Autodesk Inventor part; units mm, degrees
ref_plane "YZ Plane" through (0, 0, 0) normal (1, 0, 0) x (0, 1, 0)
ref_plane "XZ Plane" through (0, 0, 0) normal (0, 1, 0) x (-1, 0, 0)
ref_plane "XY Plane" through (0, 0, 0) normal (0, 0, 1) x (1, 0, 0)
sketch "Sketch1" plane through (0, 0, 0) normal (0, 1, 0) x (-1, 0, 0)
  line L0 (0, 0) -> (75, 0)
  line L1 (77, -2) -> (77, -75)
  line L2 (75, -77) -> (2, -77)
  line L3 (0, -75) -> (0, 0)
  line L4 (0, 0) -> (0, -8.5)
  line L5 (6, -8.5) -> (8.5, -8.5)
  line L6 (8.5, -48.5) -> (8.5, -68.5)
  circle A0 centre (8.5, -8.5) radius 2.5
  circle A1 centre (8.5, -28.5) radius 2.5
  circle A2 centre (8.5, -48.5) radius 2.5
  circle A3 centre (8.5, -68.5) radius 2.5
  line L7 (68.5, -28.5) -> (68.5, -48.5)
  line L8 (68.5, -48.5) -> (68.5, -68.5)
  line L9 (68.5, -68.5) -> (38.5, -68.5)
  circle A4 centre (38.5, -8.5) radius 2.5
  circle A5 centre (68.5, -8.5) radius 2.5
  circle A6 centre (68.5, -28.5) radius 2.5
  circle A7 centre (68.5, -48.5) radius 2.5
  circle A8 centre (68.5, -68.5) radius 2.5
  circle A9 centre (38.5, -68.5) radius 2.5
  line L10 (77, 0) -> (58.5, 0)
  line L11 (58.5, -18.5) -> (61, -18.5)
  line L12 (77, -18.5) -> (77, 0)
  line L13 (2, 0) -> (18.5, 0)
  line L14 (18.5, -8.5) -> (18.5, -18.5)
  line L15 (18.5, -18.5) -> (0, -18.5)
  line L16 (0, -18.5) -> (0, -2)
  line L17 (0, -77) -> (18.5, -77)
  line L18 (18.5, -61) -> (18.5, -58.5)
  line L19 (0, -58.5) -> (0, -77)
  circle A10 centre (58.5, -18.5) radius 2.5
  circle A11 centre (18.5, -18.5) radius 2.5
  circle A12 centre (18.5, -58.5) radius 2.5
  circle A13 centre (58.5, -58.5) radius 2.5
  line L20 (18.5, -18.5) -> (28.5, -18.5)
  line L21 (58.5, -58.5) -> (48.5, -58.5)
  circle A14 centre (28.5, -18.5) radius 2.5
  circle A15 centre (48.5, -18.5) radius 2.5
  circle A16 centre (48.5, -58.5) radius 2.5
  circle A17 centre (28.5, -58.5) radius 2.5
  line L22 (58.5, -38.5) -> (48.5, -38.5)
  line L23 (28.5, -38.5) -> (18.5, -38.5)
  circle A18 centre (58.5, -38.5) radius 2.5
  circle A19 centre (48.5, -38.5) radius 2.5
  circle A20 centre (28.5, -38.5) radius 2.5
  circle A21 centre (18.5, -38.5) radius 2.5
  circle A22 centre (38.5, -28.5) radius 2.5
  circle A23 centre (38.5, -38.5) radius 2.5
  line L24 (28.5, -58.5) -> (28.5, -38.5)
  circle A24 centre (38.5, -48.5) radius 2.5
  line L25 (36, -48.5) -> (36, -38.5)
  line L26 (41, -38.5) -> (41, -48.5)
  arc A25 (77, -2) -> (75, 0) centre (75, -2) ccw
  arc A26 (75, -77) -> (77, -75) centre (75, -75) ccw
  arc A27 (0, -75) -> (2, -77) centre (2, -75) ccw
  arc A28 (2, 0) -> (0, -2) centre (2, -2) ccw
  line L27 (68.5, -8.5) -> (68.5, -11)
  line L28 (68.5, -26) -> (68.5, -28.5)
  line L29 (58.5, 0) -> (58.5, -8.5)
  line L30 (58.5, -16) -> (58.5, -18.5)
  line L31 (38.5, -8.5) -> (41, -8.5)
  line L32 (66, -8.5) -> (68.5, -8.5)
  line L33 (58.5, -18.5) -> (58.5, -21)
  line L34 (58.5, -36) -> (58.5, -38.5)
  line L35 (58.5, -18.5) -> (56, -18.5)
  line L36 (51, -18.5) -> (48.5, -18.5)
  line L37 (48.5, -18.5) -> (46.7322, -20.2678)
  line L38 (40.2678, -26.7322) -> (28.5, -38.5)
  line L39 (28.5, -18.5) -> (40.2678, -30.2678)
  line L40 (46.7322, -36.7322) -> (48.5, -38.5)
  line L41 (48.5, -38.5) -> (46, -38.5)
  line L42 (41, -38.5) -> (28.5, -38.5)
  line L43 (48.5, -38.5) -> (46.7322, -40.2678)
  line L44 (41, -46) -> (36.7322, -50.2678)
  line L45 (30.2678, -56.7322) -> (28.5, -58.5)
  line L46 (48.5, -58.5) -> (36, -46)
  line L47 (30.2678, -40.2678) -> (28.5, -38.5)
  line L48 (18.5, -58.5) -> (21, -58.5)
  line L49 (26, -58.5) -> (28.5, -58.5)
  line L50 (18.5, -58.5) -> (16, -58.5)
  line L51 (8.5, -58.5) -> (0, -58.5)
  line L52 (8.5, -28.5) -> (8.5, -31)
  line L53 (8.5, -46) -> (8.5, -48.5)
  line L54 (8.5, -8.5) -> (8.5, -11)
  line L55 (8.5, -26) -> (8.5, -28.5)
  line L56 (8.5, -8.5) -> (11, -8.5)
  line L57 (18.5, -8.5) -> (38.5, -8.5)
  line L58 (28.5, -38.5) -> (28.5, -36)
  line L59 (28.5, -21) -> (28.5, -18.5)
  point P0 (77, -77)
  dimension "d9" = 5
  dimension "d15" = 5
  dimension "d17" = 5
  dimension "d29" = 5
  dimension "d32" = 5
  dimension "d0" = 77
  dimension "d1" = 77
  dimension "d2" = 8.5
  dimension "d3" = 8.5
  dimension "d4" = 20
  dimension "d5" = 20
  dimension "d6" = 20
  dimension "d7" = 5
  dimension "d8" = 5
  dimension "d10" = 5
  dimension "d11" = 30
  dimension "d12" = 30
  dimension "d13" = 20
  dimension "d14" = 20
  dimension "d16" = 5
  dimension "d18" = 18.5
  dimension "d19" = 18.5
  dimension "d20" = 18.5
  dimension "d21" = 18.5
  dimension "d22" = 18.5
  dimension "d23" = 18.5
  dimension "d24" = 5
  dimension "d25" = 5
  dimension "d26" = 10
  dimension "d27" = 10
  dimension "d28" = 10
  dimension "d30" = 5
  dimension "d31" = 20
  dimension "d33" = 5
  dimension "d34" = 5
  dimension "d35" = 2
  dimension "d36" = 2
extrude "Extrusion1" add sketch "Sketch1" along normal blind 6 contours L0 A25 L1 A26 L2 A27 L3 A28
sketch "Sketch2" plane through (0, 6, 0) normal (0, 1, 0) x (1, 0, 0)
  line L0 (0, 0) -> (-23.5, 0)
  line L1 (-23.5, 0) -> (-23.5, 23.5)
  line L2 (-23.5, 23.5) -> (0, 23.5)
  line L3 (0, 23.5) -> (0, 0)
  line L4 (-77, 75) -> (-77, 2)
  line L5 (-77, 67.2397) -> (-77, 80.0778)
  line L6 (-2, 77) -> (-75, 77)
  line L7 (-67.8517, 77) -> (-77, 77)
  line L8 (-77, 77) -> (-53.5, 77)
  line L9 (-53.5, 77) -> (-53.5, 53.5)
  line L10 (-53.5, 53.5) -> (-77, 53.5)
  line L11 (-77, 53.5) -> (-77, 77)
  line L12 (-51.5, 53.5) -> (-25.5, 53.5)
  line L13 (-23.5, 51.5) -> (-23.5, 25.5)
  line L14 (-25.5, 23.5) -> (-51.5, 23.5)
  line L15 (-53.5, 25.5) -> (-53.5, 51.5)
  arc A0 (-53.5, 25.5) -> (-51.5, 23.5) centre (-51.5, 25.5) ccw
  arc A1 (-25.5, 23.5) -> (-23.5, 25.5) centre (-25.5, 25.5) ccw
  arc A2 (-23.5, 51.5) -> (-25.5, 53.5) centre (-25.5, 51.5) ccw
  arc A3 (-51.5, 53.5) -> (-53.5, 51.5) centre (-51.5, 51.5) ccw
  dimension "d39" = 23.5
  dimension "d40" = 23.5
  dimension "d41" = 23.5
  dimension "d42" = 23.5
  dimension "d43" = 2
extrude "Extrusion2" cut sketch "Sketch2" against normal blind 1 contours L12 A2 L13 A1 L14 A0 L15 A3
sketch "Sketch3" plane through (0, 0, 0) normal (0, -1, 0) x (1, 0, 0)
  line L0 (-51.5, -53.5) -> (-25.5, -53.5)
  line L1 (-53.5, -25.5) -> (-53.5, -51.5)
  line L2 (-25.5, -23.5) -> (-51.5, -23.5)
  line L3 (-23.5, -51.5) -> (-23.5, -25.5)
  line L4 (-53.5, -53.5) -> (-23.5, -53.5)
  line L5 (-23.5, -53.5) -> (-23.5, -38.5)
  line L6 (-53.5, -38.5) -> (-23.5, -38.5)
  line L7 (-53.5, -38.5) -> (-53.5, -53.5)
  point P0 (0, 0)
extrude "Extrusion3" add sketch "Sketch3" along normal blind 15
sketch "Sketch4" plane through (-23.5, 0, -53.5) normal (0, 0, -1) x (-1, 0, 0)
  line L0 (2.5, 0) -> (0, 0)
  line L1 (0, 0) -> (0, -15)
  line L2 (0, -8) -> (15, -8)
  line L3 (30, 0) -> (30, -15)
  circle A0 centre (15, -8) radius 4
  line L4 (0, 0) -> (0, -15)
  line L5 (0, -8) -> (0, -15)
  line L6 (30, -15) -> (0, -15)
  point P0 (-23.5, 0)
  dimension "d49" = 15
  dimension "d50" = 8
  dimension "d53" = 7
extrude "Extrusion4" cut sketch "Sketch4" against normal blind 22
sketch "Sketch5" plane through (0, 6, 0) normal (0, 1, 0) x (1, 0, 0)
  arc A0 (-25.5, 23.5) -> (-23.5, 25.5) centre (-25.5, 25.5) ccw
  line L0 (-25.5, 23.5) -> (-51.5, 23.5)
  arc A1 (-53.5, 25.5) -> (-51.5, 23.5) centre (-51.5, 25.5) ccw
  line L1 (-53.5, 25.5) -> (-53.5, 51.5)
  arc A2 (-51.5, 53.5) -> (-53.5, 51.5) centre (-51.5, 51.5) ccw
  line L2 (-51.5, 53.5) -> (-25.5, 53.5)
  arc A3 (-23.5, 51.5) -> (-25.5, 53.5) centre (-25.5, 51.5) ccw
  line L3 (-23.5, 51.5) -> (-23.5, 25.5)
  arc A4 (0, 75) -> (-2, 77) centre (-2, 75) ccw
  line L4 (-2, 77) -> (-75, 77)
  arc A5 (-75, 77) -> (-77, 75) centre (-75, 75) ccw
  line L5 (-77, 75) -> (-77, 2)
  arc A6 (-77, 2) -> (-75, 0) centre (-75, 2) ccw
  line L6 (-75, 0) -> (-2, 0)
  arc A7 (-2, 0) -> (0, 2) centre (-2, 2) ccw
  line L7 (0, 2) -> (0, 75)
  circle A8 centre (-58.5, 38.5) radius 2.5
  circle A9 centre (-68.5, 28.5) radius 2.5
  circle A10 centre (-68.5, 48.5) radius 2.5
  circle A11 centre (-68.5, 68.5) radius 2.5
  circle A12 centre (-8.5, 48.5) radius 2.5
  circle A13 centre (-8.5, 68.5) radius 2.5
  circle A14 centre (-18.5, 38.5) radius 2.5
  circle A15 centre (-28.5, 58.5) radius 2.5
  circle A16 centre (-58.5, 58.5) radius 2.5
  circle A17 centre (-48.5, 58.5) radius 2.5
  circle A18 centre (-28.5, 18.5) radius 2.5
  circle A19 centre (-38.5, 8.5) radius 2.5
  circle A20 centre (-18.5, 18.5) radius 2.5
  circle A21 centre (-18.5, 58.5) radius 2.5
  circle A22 centre (-58.5, 18.5) radius 2.5
  circle A23 centre (-8.5, 28.5) radius 2.5
  circle A24 centre (-8.5, 8.5) radius 2.5
  circle A25 centre (-68.5, 8.5) radius 2.5
  circle A26 centre (-38.5, 68.5) radius 2.5
  circle A27 centre (-48.5, 18.5) radius 2.5
  point P0 (0, 0)
properties part number "piezamovil"
Read the model definition and answer for the solid it produces. Units are mm, in the model's axes. A direction names the side the tool comes from. Give positions to 0.01 mm unless a question says otherwise; leave off trailing zeros. Loops run counter-clockwise (first coordinate to the right, second up) from the corner with the lowest first, then second, coordinate; pieces in that order, holes last. Notation, with made-up numbers: M -26,58.5 L 5,58.5 A18 cw 5,81.5 Z; hole C -21,-9.5 d7. An arc over 180 degrees is marked long. Write each question's results on one line, items separated by ' | '.
1. Section C-C on x = -68.5 is taken. Give the vertices of the cut face in (y, z), plus the area to 3 significant figures.
Values:
outline: M 0,-77 L 6,-77 L 6,-71 L 0,-71 Z; M 0,-66 L 6,-66 L 6,-51 L 0,-51 Z; M 0,-46 L 6,-46 L 6,-31 L 0,-31 Z; M 0,-26 L 6,-26 L 6,-11 L 0,-11 Z; M 0,-6 L 6,-6 L 6,0 L 0,0 Z | area: 342 mm^2
2. Section B-B on y = -8 is taken. Give the vertices of the cut face in (x, z), plus the area to 3 significant figures.
Values:
outline: M -53.5,-53.5 L -42.5,-53.5 L -42.5,-38.5 L -53.5,-38.5 Z; M -34.5,-53.5 L -23.5,-53.5 L -23.5,-38.5 L -34.5,-38.5 Z | area: 330 mm^2
3. Given pin 1 (2 mm diameter, centred on x = -31, z = -17.5, fed in from -Y); pin 2 (4.5 mm diameter, centred on x = -38.5, z = -28.5, fed in from +Y); pin 3 (4.5 mm diameter, centred on x = -40.5, y = -5, fed in from +Z); pin 4 (4 mm diameter, centred on x = -40.5, z = -28, fed in from +Y), each flat-ended and moving along its own axis, determine where each tip first touches the part or whether it passes through.
Values:
pin 1: stops at y = 0 | pin 2: passes through | pin 3: stops at z = -38.5 | pin 4: stops at y = 5
4. Section A-A on x = -58.5 is taken. Give the vertices of the cut face in (y, z).
Values:
outline: M 0,-77 L 6,-77 L 6,-61 L 0,-61 Z; M 0,-56 L 6,-56 L 6,-41 L 0,-41 Z; M 0,-36 L 6,-36 L 6,-21 L 0,-21 Z; M 0,-16 L 6,-16 L 6,0 L 0,0 Z
5. A tool of negligible diameter and unlimited length cuts with its end or side. For faces 4 (the face through (-24.1, 5.51, -24.07)), 5 (the face through (-53.5, -7, -46)), 6 (the face through (-66.06, 2.96, -69.04)), from which of +Z, -Z, +X, -X, +Y, -Y can it reach the whole face along a straight path? Write none if from no direction.
Values:
face 4: +Y | face 5: +Z, -Z, -X, -Y | face 6: +Y, -Y
6. The mould has two halves that part along X. Classify faces 1 (the face through (0, 3, -39)), 2 (the face through (-40.81, 2.96, -67.54)), 3 (the face through (-76.4, 2.96, -0.57)): pulls with the +X half, pulls with the -X half, needs draft (parallel to the pull), parting line crosses it, or undercut.
Values:
face 1: pulls with the +X half | face 2: undercut | face 3: pulls with the -X half
7. Straight lines are drawn through the part: line 1 (X direction, y = 3.1, z = -58.5); line 2 (X direction, y = 1.4, z = -48.5); line 3 (Z direction, x = -38.5, y = 1.25). For each, find the intervals that lie inside material, in ascending order. Write a range as [from, to].
Values:
line 1: x = [-77, -61], [-56, -51], [-46, -31], [-26, -21], [-16, 0] | line 2: x = [-77, -71], [-66, -41], [-36, -11], [-6, 0] | line 3: z = [-77, -71], [-66, -51], [-36, -31], [-26, -11], [-6, 0]
8. Section D-D on z = -28.5 is taken. Give the vertices of the cut face in (x, y), plus the area to 3 significant figures.
Values:
outline: M -77,0 L -71,0 L -71,6 L -77,6 Z; M -66,0 L -41,0 L -41,5 L -53.5,5 L -53.5,6 L -66,6 Z; M -36,0 L -11,0 L -11,6 L -23.5,6 L -23.5,5 L -36,5 Z; M -6,0 L 0,0 L 0,6 L -6,6 Z | area: 347 mm^2
